from build123d import *

# Parameters (mm, degrees)
F0_R     = 12.5
F1_DEPTH = 310
F2_R     = 6
F3_DEPTH = 45
F4_SIZE  = 1
F5_R     = 20.961122
F5_R_2   = 10
F6_DEPTH = 160


with BuildPart() as f1:
    # F0 (on Front) → F1 (new body)
    with BuildSketch(Plane.XZ):
        Circle(F0_R)
    extrude(amount=F1_DEPTH)

    # F2 (on face) → F3 (cut)
    with BuildSketch(Plane(origin=(0, 0, 0), x_dir=(-1, 0, 0), z_dir=(0, 1, 0))):
        Circle(F2_R)
    extrude(amount=-F3_DEPTH, mode=Mode.SUBTRACT)

    # F4
    f4_edges = [f1.edges().sort_by_distance(p)[0] for p in [
        (-12.5, 0, 0),
    ]]
    chamfer(f4_edges, length=F4_SIZE)

    # F5 (on Front) → F6 (cut)
    with BuildSketch(Plane.XZ):
        Circle(F5_R)
        Circle(F5_R_2, mode=Mode.SUBTRACT)
    extrude(amount=F6_DEPTH, mode=Mode.SUBTRACT)


solid = f1.part
Source: CAD feature listing. Evaluate the final solid. Frame: model axes, mm. A direction names the side the tool comes from. Round coordinates to 2 decimals unless told otherwise and drop trailing zeros. Write each loop counter-clockwise with the first axis right and the second up, starting at its lowest first coordinate (ties: lowest second). Pieces come first, ordered by that corner, then holes. Notation, with made-up numbers: M -18.5,41 L 33.5,41 A18 cw 33.5,58 Z; hole C 48,26.5 d2. An arc over 180 degrees is marked long. One line per item, written item: value. Start each with the question number.
Item 1: Mould query, pull axis X, two halves, no side actions, for faces 3 (the cylindrical face through (-2.17, -78.88, -9.76)), 4 (the flat face through (0, -45, 0)), 5 (the flat face through (0, -310, 0)). Classes: pulls with the +X half, pulls with the -X half, needs draft (parallel to the pull), parting line crosses it, or undercut.
Item 2: Pin query (flat end, axial travel): pin 1 (8 mm diameter, centred on y = -132, z = -8, fed in from -X); pin 2 (6 mm diameter, centred on y = -165, z = -7.5, fed in from -X); pin 3 (6 mm diameter, centred on y = -61.5, z = -9.5, fed in from -X). Return the tip coordinate at first contact, or that it passes through.
Item 3: Section query D-D (y = -254.5). Return the cut outline in (x, z), plus the area to 3 significant figures.
Item 4: Section query C-C (y = -74.5). Return the cut outline in (x, z).
Item 5: Ray query, L1, parallel to Z at x = 0, y = -13.5; L2, parallel to Y at x = -2, z = 0.5; L3, parallel to Y at x = 3.75, z = 10. Return the intervals inside material, ascending. Write a range as from..to.
Item 6: Section query A-A (z = 0). Return the cut outline in (x, y).
Item 7: Set-up query: faces 1 (the flat face through (0, 0, -7)), 2 (the flat face through (-0.1, -160, 10.2)). Return all of +Z, -Z, +X, -X, +Y, -Y with unobstructed straight access to the full face (end or side cutting, diameter ignored); none if empty.
Item 8: Section query B-B (x = 0). Return the cut outline in (y, z).
Result set:
1. face 3: parting line crosses it
1. face 4: undercut
1. face 5: needs draft
2. pin 1: stops at x = -9.17
2. pin 2: stops at x = -11.66
2. pin 3: stops at x = -7.6
3. outline: C 0,0 d25
3. area: 491 mm²
4. outline: C 0,0 d20
5. L1: z = -10..-6, 6..10
5. L2: y = -310..-45
5. L3: y = -310..-160
6. outline: M -12.5,-310 L 12.5,-310 L 12.5,-160 L 10,-160 L 10,0 L 6,0 L 6,-45 L -6,-45 L -6,0 L -10,0 L -10,-160 L -12.5,-160 Z
7. face 1: +Z, -Z, +X, -X, +Y
7. face 2: +Y
8. outline: M -310,-12.5 L -160,-12.5 L -160,-10 L 0,-10 L 0,-6 L -45,-6 L -45,6 L 0,6 L 0,10 L -160,10 L -160,12.5 L -310,12.5 Z
